Autodesk Inventor part; units mm, degrees
ref_plane "YZ Plane" through (0, 0, 0) normal (1, 0, 0) x (0, 1, 0)
ref_plane "XZ Plane" through (0, 0, 0) normal (0, 1, 0) x (-1, 0, 0)
ref_plane "XY Plane" through (0, 0, 0) normal (0, 0, 1) x (1, 0, 0)
sketch "Sketch1" plane through (0, 0, 0) normal (0, 1, 0) x (-1, 0, 0)
  line L0 (0, 0) -> (870, 0)
  line L1 (870, 0) -> (870, 870)
  line L2 (870, 870) -> (0, 870)
  line L3 (0, 870) -> (0, 0)
  dimension "d0" = 870
  dimension "d1" = 870
extrude "Extrusion1" add sketch "Sketch1" along normal blind 30
sketch "Sketch2" plane through (0, 0, 0) normal (0, -1, 0) x (1, 0, 0)
  line L0 (0, 0) -> (-870, 0)
  line L1 (0, 870) -> (0, 0)
  line L2 (-870, 870) -> (0, 870)
  line L3 (-870, 0) -> (-870, 870)
  line L4 (-10, 860) -> (-10, 10)
  line L5 (-10, 10) -> (-860, 10)
  line L6 (-860, 10) -> (-860, 860)
  line L7 (-860, 860) -> (-10, 860)
  dimension "d4" = 10
extrude "Extrusion2" cut sketch "Sketch2" against normal blind 27.5 contours L4 L5 L6 L7
sketch "Sketch3" plane through (0, 30, 0) normal (0, 1, 0) x (1, 0, 0)
  circle A0 centre (-435, -435) radius 73.66
  line L0 (0, 0) -> (-870, 0)
  line L1 (-870, 0) -> (-870, -870)
  line L2 (-870, -870) -> (0, -870)
  line L3 (0, -870) -> (0, 0)
  line L4 (-435, 0) -> (-435, -870) construction
  line L5 (-870, -435) -> (0, -435) construction
  point P0 (-435, -435)
  dimension "d7" = 147.32
extrude "Extrusion3" cut sketch "Sketch3" against normal blind 25.4 contours A0
properties part number "housingLid" material "Steel, Galvanized"
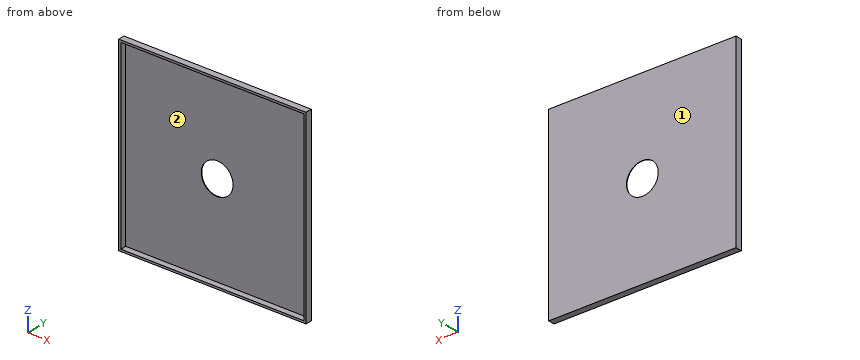
Part model, mm, in its own coordinate system. Face numbers are marked on the shaded views. Coordinates: 2 decimals unless noted, no trailing zeros. Loops run counter-clockwise (first coordinate to the right, second up) from the corner with the lowest first, then second, coordinate; pieces in that order, holes last. Notation, with made-up numbers: M 1,61 L 54,61 A25 ccw 54,98 Z; hole C 77,22 d9. An arc over 180 degrees is marked long. Use a Markdown table: item, result. Add a question column.
Q1. Cut at C-C (y = 6.5). Write the cut outline in (x, z), and give its area (3 significant figures).
Q2. Mould opens along Z. For the marked faces 1 and 2 say: +Z half, -Z half, draft (parallel to the pull), parting line (faces both ways), or undercut.
Q3. Cut at A-A (z = 435). Write the cut outline in (x, y).
Q4. Probe L1, parallel to X at y = 18.5, z = 810; L2, parallel to Z at x = -394.5, y = 12.25; L3, parallel to X at y = 28.15, z = 435. List the from-to ranges inside material, lowest first.
Q5. Pin check, flat tip, straight feed: P1, Ø1, axis at x = -512, z = 634, coming from the -Y side. Stop position of the tip, or through.
Q6. Cut at B-B (x = -458.5). Write the cut outline in (y, z), and give its area (3 significant figures).
Q7. Cut at D-D (x = -307.5). Write the cut outline in (y, z).
Worked out:
| question | item | result |
|---|---|---|
| 1 | outline | M -870,0 L 0,0 L 0,870 L -870,870 Z; hole M -860,10 L -10,10 L -10,860 L -860,860 Z |
| 1 | area | 34,400 mm2 |
| 2 | face 1 | draft |
| 2 | face 2 | undercut |
| 3 | outline | M -870,0 L -860,0 L -860,27.5 L -508.66,27.5 L -508.66,30 L -870,30 Z; M -361.34,27.5 L -10,27.5 L -10,0 L 0,0 L 0,30 L -361.34,30 Z |
| 4 | L1 | x = -870 to -860, -10 to 0 |
| 4 | L2 | z = 0 to 10, 860 to 870 |
| 4 | L3 | x = -870 to -508.66, -361.34 to 0 |
| 5 | P1 | stops at y = 27.5 |
| 6 | outline | M 0,0 L 30,0 L 30,365.19 L 27.5,365.19 L 27.5,10 L 0,10 Z; M 0,860 L 27.5,860 L 27.5,504.81 L 30,504.81 L 30,870 L 0,870 Z |
| 6 | area | 2,380 mm2 |
| 7 | outline | M 0,0 L 30,0 L 30,870 L 0,870 L 0,860 L 27.5,860 L 27.5,10 L 0,10 Z |
